Verification items for the finished model (mm, model axes). A direction names the side the tool comes from. Round coordinates to 2 decimals unless told otherwise and drop trailing zeros. Write each loop counter-clockwise with the first axis right and the second up, starting at its lowest first coordinate (ties: lowest second). Pieces come first, ordered by that corner, then holes. Notation, with made-up numbers: M 83.25,51 L 88.25,51 A26 ccw 88.25,85 Z; hole C 80.5,-34.5 d6. An arc over 180 degrees is marked long. Answer in a Markdown table with one row per item. Add a question column.
1. Sectioned sample at A-A on z = 2.1. Record the cut outline in (x, y).
2. Set-up check for faces 5 (the flat face through (0, -35.418, 3)), 6 (the flat face through (2.48, -1.35, 1.23)): record each of +Z, -Z, +X, -X, +Y, -Y from which the full face is reachable in a straight line by a thin tool's end or side.
3. Sectioned sample at B-B on x = 0. Record the cut outline in (y, z), plus the area to 3 significant figures.
4. Draft check along Y on faces 1 (the flat face through (-7.543, -18, 3)), 2 (the cylindrical face through (-0.21, 7.58, 2.71)), 3 (the cylindrical face through (1.39, 0.53, 3.98)), 4 (the flat face through (0, 2.983, 1)). Enter one of: pulls with the +Y half, pulls with the -Y half, needs draft (parallel to the pull), parting line crosses it, or undercut.
5. Sectioned sample at C-C on y = -1. Record the cut outline in (x, z).
6. Go/stop test with flat-tipped pins: pin 1 Ø1.5 at (x, z) = (2, 1.5) entering from +Y; pin 2 Ø1 at (x, z) = (5, 1) entering from +Y. Record where each tip stops, or that it passes through.
7. Sectioned sample at D-D on x = 2.25. Record the cut outline in (y, z), plus the area to 3 significant figures.
8. Material ranges on probe 1 along X at (y, z) = (0.5, 2.6); probe 2 along Y at (x, z) = (-2, 2.2); probe 3 along Y at (x, z) = (1.5, 2.15), recorded low to high.
```python
from build123d import *
from build123d.topology import SkipClean

# Parameters (mm, degrees)
BOSS_EXTRUDE1_DEPTH = 2.5
SKETCH3_R           = 1.5
BOSS_EXTRUDE2_DEPTH = 3


with BuildPart() as part:
    # Sketch1 → Boss-Extrude1 (new body)
    # profile 1 of 2: a face of its own
    with BuildSketch(Plane.XY):
        with BuildLine():
            ThreePointArc((-7.542881817, 0.082245335), (-0.042881817, -7.417754665), (7.457118183, 0.082245335))
            ThreePointArc((7.457118183, 0.082245335), (-0.042881817, 7.582245335), (-7.542881817, 0.082245335))
        make_face()
        Polygon((1.632118183, 2.983430437), (3.307118183, 0.082245335), (1.632118183, -2.818939768), (-0.042881817, -2.818939768), (-1.717881817, -2.818939768), (-3.392881817, 0.082245335), (-1.717881817, 2.983430437), (-0.042881817, 2.983430437), align=None, mode=Mode.SUBTRACT)
    # profile 2 of 2: a face of its own
    with BuildSketch(Plane.XY):
        with BuildLine():
            Line((7.457118183, -35.417754665), (7.457118183, 0.082245335))
            ThreePointArc((7.457118183, 0.082245335), (-0.042881817, -7.417754665), (-7.542881817, 0.082245335))
            Line((-7.542881817, 0.082245335), (-7.542881817, -35.417754665))
            Line((-7.542881817, -35.417754665), (7.457118183, -35.417754665))
        make_face()
    extrude(amount=BOSS_EXTRUDE1_DEPTH)

    # Sketch3 → Boss-Extrude2 (add)
    with SkipClean():  # the faces are left unmerged after this step: merging them gives an invalid solid
        with BuildSketch(Plane.XY.offset(2.5)):
            with BuildLine():
                Line((7.457118183, 0.082245335), (7.457118183, -35.417754665))
                Line((7.457118183, -35.417754665), (-7.542881817, -35.417754665))
                Line((-7.542881817, -35.417754665), (-7.542881817, 0.082245335))
                ThreePointArc((-7.542881817, 0.082245335), (-0.042881817, 7.582245335), (7.457118183, 0.082245335))
            make_face()
            with Locations((-0.042881817, 0.082245335)):
                Circle(SKETCH3_R, mode=Mode.SUBTRACT)
        extrude(amount=BOSS_EXTRUDE2_DEPTH)
    add(part.part.scale(1), mode=Mode.REPLACE)  # the faces are merged on a copy


solid = part.part
```
Geometry check:
| question | item | result |
|---|---|---|
| 1 | outline | M -7.54,-35.42 L 7.46,-35.42 L 7.46,0.08 A7.5 ccw -7.54,0.08 Z; hole M -3.39,0.08 L -1.72,-2.82 L 1.63,-2.82 L 3.31,0.08 L 1.63,2.98 L -1.72,2.98 Z |
| 2 | face 5 | +Z, -Z, +X, -X, -Y |
| 2 | face 6 | -Z |
| 3 | outline | M -35.42,0 L -2.82,0 L -2.82,2.5 L -1.42,2.5 L -1.42,5.5 L -35.42,5.5 Z; M 1.58,2.5 L 2.98,2.5 L 2.98,0 L 7.58,0 L 7.58,5.5 L 1.58,5.5 Z |
| 3 | area | 213 mm2 |
| 4 | face 1 | needs draft |
| 4 | face 2 | pulls with the +Y half |
| 4 | face 3 | undercut |
| 4 | face 4 | undercut |
| 5 | outline | M -7.54,0 L -2.77,0 L -2.77,2.5 L -1.08,2.5 L -1.08,5.5 L -7.54,5.5 Z; M 1,2.5 L 2.68,2.5 L 2.68,0 L 7.46,0 L 7.46,5.5 L 1,5.5 Z |
| 6 | pin 1 | stops at y = 7.47 |
| 6 | pin 2 | stops at y = 6.05 |
| 7 | outline | M -35.42,0 L -1.75,0 L -1.75,2.5 L 1.91,2.5 L 1.91,0 L 7.22,0 L 7.22,5.5 L -35.42,5.5 Z |
| 7 | area | 225 mm2 |
| 8 | probe 1 | x = -7.53 to -1.48, 1.4 to 7.45 |
| 8 | probe 2 | y = -35.42 to -2.33, 2.49 to 7.32 |
| 8 | probe 3 | y = -35.42 to -2.82, 2.98 to 7.42 |
